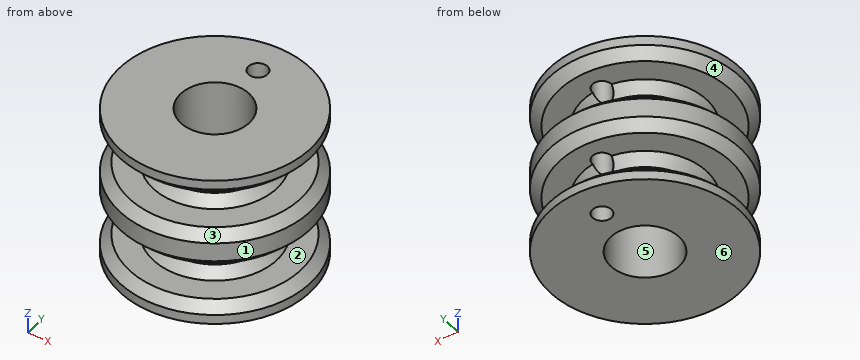
Autodesk Inventor part; units mm, degrees
ref_plane "YZ Plane" through (0, 0, 0) normal (1, 0, 0) x (0, 1, 0)
ref_plane "XZ Plane" through (0, 0, 0) normal (0, 1, 0) x (-1, 0, 0)
ref_plane "XY Plane" through (0, 0, 0) normal (0, 0, 1) x (1, 0, 0)
sketch "Sketch1" plane through (0, 0, 0) normal (0, 0, 1) x (1, 0, 0)
  circle A0 centre (0, 0) radius 5
  dimension "d0" = 10
extrude "Extrusion1" add sketch "Sketch1" along normal blind 8
ref_plane "Work Plane2" through (0, 0, 6) normal (0, 0, 1) x (1, 0, 0)
ref_plane "Work Plane1" through (0, 0, 4) normal (0, 0, 1) x (1, 0, 0)
sketch "Sketch2" plane through (0, 0, 6) normal (0, 0, 1) x (1, 0, 0)
  circle A0 centre (0, 0) radius 5
  circle A1 centre (0, 0) radius 2.75
  dimension "d3" = 5.5
  dimension "d4" = 10
extrude "Extrusion2" cut sketch "Sketch2" along normal mid plane 2
mirror "Mirror1" about plane through (0, 0, 4) normal (0, 0, 1) of "Extrusion2"
sketch "Sketch3" plane through (0, 0, 0) normal (0, 0, -1) x (-1, 0, 0)
  point P0 (0, 0)
sketch "Sketch4" plane through (0, 0, 0) normal (0, 0, -1) x (-1, 0, 0)
  circle A0 centre (0, 0) radius 1.8
  dimension "d11" = 3.6
extrude "Extrusion3" cut sketch "Sketch4" against normal blind 10
sketch "Sketch5" plane through (0, 0, 8) normal (0, 0, 1) x (1, 0, 0)
  circle A0 centre (0, 3.2193) radius 0.5
  point P0 (0, 0)
  dimension "d14" = 1
extrude "Extrusion4" cut sketch "Sketch5" against normal blind 10
chamfer "Chamfer1" distance 0.5 angle 45 12 edges at (2.0001, 1.8873, 7) (-1.8873, -2.0001, 7) (2.0001, 1.8873, 5) (-1.8873, -2.0001, 5) (2.0001, 1.8873, 3) (-1.8873, -2.0001, 3) (2.0001, 1.8873, 1) (-1.8873, -2.0001, 1) (-5, 0, 7) (-5, 0, 5) (-5, 0, 1) (-5, 0, 3)
properties part number "MotorPullyRounded"
Source: CAD feature listing. Evaluate the final solid. Frame: model axes, mm. Face numbers are marked on the shaded views. A direction names the side the tool comes from. Give positions to 0.01 mm unless a question says otherwise; leave off trailing zeros. Order: outer loops, then holes, each group sorted by start corner. A loop starts at its lowest first (then second) coordinate and runs counter-clockwise, first axis right, second up. Notation, with made-up numbers: (67.25, 7.25) -> (73.25, 7.25) arc R21 ccw to (73.25, 37.25) -> close; hole circle Ø4 at (-39, 35.25). An arc over 180 degrees is marked (long way). Write item = value, one per line.
Item 1: Section query A-A (y = -3.5). State how many separate pieces and enclosed holes the cut face has, then the cut area to 3 significant figures.
Check result:
separate_pieces = 3
enclosed_holes = 0
area = 27.1 mm²
Item 2: Section query C-C (z = 1.75). Output: boundary loops of the cut face in (x, y), then the cut area to 3 significant figures.
Check result:
outline = (-0.16, 2.75) arc R2.75 ccw (long way) to (0.16, 2.75) arc R0.5 cw to start; hole circle Ø3.6 at (0, 0)
area = 13.6 mm²
Item 3: Set-up query: the marked faces 1 and 2. Return all of +Z, -Z, +X, -X, +Y, -Y with unobstructed straight access to the full face (end or side cutting, diameter ignored); none if empty.
Check result:
face_1 = +Z, -Z
face_2 = none
Item 4: Mould query, pull axis Z, two halves, no side actions, for the marked faces 3, 4, 5 and 6. Classes: +Z half, -Z half, draft (parallel to the pull), parting line (faces both ways), or undercut.
Check result:
face_3 = undercut
face_4 = undercut
face_5 = draft
face_6 = -Z half
Item 5: Contact query for flat-ended pins moving along their axis: pin 1 (1 mm diameter, centred on x = 0.5, z = 6, fed in from -Y); pin 2 (1.5 mm diameter, centred on y = 0.5, z = 2, fed in from +X); pin 3 (1.5 mm diameter, centred on x = 0, z = 6.5, fed in from -Y). Output: stop coordinate, or through.
Check result:
pin_1 = -2.75
pin_2 = 2.97
pin_3 = -4.75
Item 6: Ray query, probe 1 along Y at (x, z) = (0, 4); probe 2 along Z at (x, y) = (-4, -1.75); probe 3 along Z at (x, y) = (-3, 3.5). Return the intervals inside material, ascending.
Check result:
probe_1 = -5 to -1.8, 1.8 to 2.72, 3.72 to 5
probe_2 = 0 to 1, 3 to 5, 7 to 8
probe_3 = 0 to 0.89, 3.11 to 4.89, 7.11 to 8
